```python
from build123d import *

# Parameters (mm, degrees)
BOSS_EXTRUDE1_DEPTH = 2.8
FILLET1_R           = 1
FILLET2_R           = 1
FILLET3_R           = 1
FILLET4_R           = 1
BOSS_EXTRUDE2_DEPTH = 1
BOSS_EXTRUDE3_DEPTH = 6.7
BOSS_EXTRUDE4_DEPTH = 1
BOSS_EXTRUDE5_DEPTH = 2.8


with BuildPart() as part:
    # Sketch1 → Boss-Extrude1 (new body)
    with BuildSketch(Plane(origin=(0, 0, 0), x_dir=(1, 0, 0), z_dir=(0, 1, 0))):
        with BuildLine():
            Line((-0.8, -0.8), (-0.8, -2.102974084))
            ThreePointArc((-0.8, -2.102974084), (0, -2.25), (0.8, -2.102974084))
            Line((0.8, -2.102974084), (0.8, -0.8))
            Line((0.8, -0.8), (2.102974084, -0.8))
            ThreePointArc((2.102974084, -0.8), (2.25, 0), (2.102974084, 0.8))
            Line((2.102974084, 0.8), (0.8, 0.8))
            Line((0.8, 0.8), (0.8, 2.102974084))
            ThreePointArc((0.8, 2.102974084), (0, 2.25), (-0.8, 2.102974084))
            Line((-0.8, 2.102974084), (-0.8, 0.8))
            Line((-0.8, 0.8), (-2.102974084, 0.8))
            ThreePointArc((-2.102974084, 0.8), (-2.25, 0), (-2.102974084, -0.8))
            Line((-2.102974084, -0.8), (-0.8, -0.8))
        make_face()
    extrude(amount=BOSS_EXTRUDE1_DEPTH)

    # Fillet1
    fillet1_edges = [part.edges().sort_by_distance(p)[0] for p in [
        (-2.25, 0, 0),
    ]]
    fillet(fillet1_edges, radius=FILLET1_R)

    # Fillet2
    fillet2_edges = [part.edges().sort_by_distance(p)[0] for p in [
        (0, 0, 2.25),
    ]]
    fillet(fillet2_edges, radius=FILLET2_R)

    # Fillet3
    fillet3_edges = [part.edges().sort_by_distance(p)[0] for p in [
        (2.25, 0, 0),
    ]]
    fillet(fillet3_edges, radius=FILLET3_R)

    # Fillet4
    fillet4_edges = [part.edges().sort_by_distance(p)[0] for p in [
        (0, 0, -2.25),
    ]]
    fillet(fillet4_edges, radius=FILLET4_R)

    # Sketch3 → Boss-Extrude2 (add)
    with BuildSketch(Plane(origin=(0, 2.8, 0), x_dir=(1, 0, 0), z_dir=(0, 1, 0))):
        Polygon((-0.583389757, 0.556274706), (-0.583389757, 1.85), (0.583389757, 1.85), (0.583389757, 0.556274706), (1.85, 0.556274706), (1.85, -0.556274706), (0.583389757, -0.556274706), (0.583389757, -1.85), (-0.583389757, -1.85), (-0.583389757, -0.556274706), (-1.85, -0.556274706), (-1.85, 0.556274706), align=None)
    extrude(amount=BOSS_EXTRUDE2_DEPTH)

    # Sketch11 → Boss-Extrude3 (add)
    with BuildSketch(Plane(origin=(0, 3.8, 0), x_dir=(1, 0, 0), z_dir=(0, 1, 0))):
        with BuildLine():
            Line((-0.799009338, -0.800292793), (-0.799009338, -2.103266877))
            ThreePointArc((-0.799009338, -2.103266877), (0.000990662, -2.250292793), (0.800990662, -2.103266877))
            Line((0.800990662, -2.103266877), (0.800990662, -0.800292793))
            Line((0.800990662, -0.800292793), (2.103964747, -0.800292793))
            ThreePointArc((2.103964747, -0.800292793), (2.250990662, -0.000292793), (2.103964747, 0.799707207))
            Line((2.103964747, 0.799707207), (0.800990662, 0.799707207))
            Line((0.800990662, 0.799707207), (0.800990662, 2.102681291))
            ThreePointArc((0.800990662, 2.102681291), (0.000990662, 2.249707207), (-0.799009338, 2.102681291))
            Line((-0.799009338, 2.102681291), (-0.799009338, 0.799707207))
            Line((-0.799009338, 0.799707207), (-2.101983422, 0.799707207))
            ThreePointArc((-2.101983422, 0.799707207), (-2.249009338, -0.000292793), (-2.101983422, -0.800292793))
            Line((-2.101983422, -0.800292793), (-0.799009338, -0.800292793))
        make_face()
    extrude(amount=BOSS_EXTRUDE3_DEPTH)

    # Sketch12 → Boss-Extrude4 (add)
    with BuildSketch(Plane(origin=(0, 10.5, 0), x_dir=(1, 0, 0), z_dir=(0, 1, 0))):
        Polygon((0.567460326, 0.546772752), (1.85, 0.546772752), (1.85, -0.562668947), (0.567460326, -0.562668947), (0.567460326, -1.850285006), (-0.565476617, -1.850285006), (-0.565476617, -0.562668947), (-1.85, -0.562668947), (-1.85, 0.546772752), (-0.565476617, 0.546772752), (-0.565476617, 1.849714994), (0.567460326, 1.849714994), align=None)
    extrude(amount=BOSS_EXTRUDE4_DEPTH)

    # Sketch13 → Boss-Extrude5 (add)
    with BuildSketch(Plane(origin=(0, 11.5, 0), x_dir=(1, 0, 0), z_dir=(0, 1, 0))):
        with BuildLine():
            Line((-0.806071321, -0.793579744), (-0.806071321, -2.096553829))
            ThreePointArc((-0.806071321, -2.096553829), (-0.006071321, -2.243579744), (0.793928679, -2.096553829))
            Line((0.793928679, -2.096553829), (0.793928679, -0.793579744))
            Line((0.793928679, -0.793579744), (2.096902763, -0.793579744))
            ThreePointArc((2.096902763, -0.793579744), (2.243928679, 0.006420256), (2.096902763, 0.806420256))
            Line((2.096902763, 0.806420256), (0.793928679, 0.806420256))
            Line((0.793928679, 0.806420256), (0.793928679, 2.10939434))
            ThreePointArc((0.793928679, 2.10939434), (-0.006071321, 2.256420256), (-0.806071321, 2.10939434))
            Line((-0.806071321, 2.10939434), (-0.806071321, 0.806420256))
            Line((-0.806071321, 0.806420256), (-2.109045406, 0.806420256))
            ThreePointArc((-2.109045406, 0.806420256), (-2.256071321, 0.006420256), (-2.109045406, -0.793579744))
            Line((-2.109045406, -0.793579744), (-0.806071321, -0.793579744))
        make_face()
    extrude(amount=BOSS_EXTRUDE5_DEPTH)


solid = part.part
```
Model file for the job. Use its own axes, mm. A direction names the side the tool comes from. Coordinates: 2 decimals unless noted, no trailing zeros. Write each loop counter-clockwise with the first axis right and the second up, starting at its lowest first coordinate (ties: lowest second). Pieces come first, ordered by that corner, then holes. Notation, with made-up numbers: (-21.75, 49) - (-4.75, 49) arc R27 ccw to (-4.75, 67) - close; hole circle Ø4 at (-8.5, 54). An arc over 180 degrees is marked (long way). One line per item, written item: value. Start each with the question number.
1. Probe line 1 (Z direction, x = 1.75, y = 3.75); line 2 (Z direction, x = 1.95, y = 5.25). List the from-to ranges inside material, lowest first. Write a range as from..to.
2. Flat gauge pins, fed straight in: pin 1 (0.8 mm diameter, centred on x = -1, y = 3, fed in from +Z); pin 2 (1 mm diameter, centred on y = 1, z = 1, fed in from +X); pin 3 (2.5 mm diameter, centred on x = 0, z = 0.5, fed in from -Y); pin 4 (0.5 mm diameter, centred on y = 11, z = -1, fed in from -X). Where does each tip first touch, or does it go through?
3. Slice it at A-A (y = 7.5). Write the cut outline in (x, z), plus the area to 3 significant figures.
4. Tool access for faces 3 (the flat face through (0.801, 7, -1)), 4 (the flat face through (-1, 7, 0.8)), 5 (the flat face through (-1, 13, -0.806)), 6 (the flat face through (0.567, 11, 1)): list every direction of +Z, -Z, +X, -X, +Y, -Y with a clear straight run to the whole face (end or side of a thin tool).
5. Mould opens along Y. For faces 1 (the flat face through (1, 11, -0.547)), 2 (the flat face through (-0.806, 13, 1)) say: released by +Y, released by -Y, zero draft, split by the parting line, or undercut.
Answers below:
1. line 1: z = -0.56..0.56
1. line 2: z = -0.8..0.8
2. pin 1: stops at z = 2.15
2. pin 2: stops at x = 2.19
2. pin 3: stops at y = 0
2. pin 4: stops at x = -0.57
3. outline: (-2.1, -0.8) - (-0.8, -0.8) - (-0.8, -2.1) arc R2.25 ccw to (0.8, -2.1) - (0.8, -0.8) - (2.1, -0.8) arc R2.25 ccw to (2.1, 0.8) - (0.8, 0.8) - (0.8, 2.1) arc R2.25 ccw to (-0.8, 2.1) - (-0.8, 0.8) - (-2.1, 0.8) arc R2.25 ccw to start
3. area: 11.5 mm^2
4. face 3: -Z, +X, +Y, -Y
4. face 4: +Z, -X, +Y, -Y
4. face 5: -Z, -X, +Y, -Y
4. face 6: +Z, +X
5. face 1: undercut
5. face 2: zero draft
